```python
from build123d import *

# Parameters (mm, degrees)
F0_W      = 25.4
F0_H      = 76.2
F3_R      = 6.35
F4_DEPTH  = 50.8
F5_R      = 76.2
F7_R      = 152.4
F10_DEPTH = 25.4
F11_COUNT = 4


with BuildPart() as f1:
    # F0 (on Front) → F1 (revolve)
    with BuildSketch(Plane.XZ):
        with Locations((-139.7, 63.5)):
            Rectangle(F0_W, F0_H)
        Polygon((-152.4, 0), (0, 0), (0, 25.4), (-127, 25.4), (-152.4, 25.4), align=None)
    revolve(axis=Axis((0, 0, 12.7), (0, 0, 1)))

    # F3 (on offset) → F4 (cut)
    with BuildSketch(Plane.XZ.offset(152.4)):
        with Locations((0, 50.8)):
            Circle(F3_R)
    extrude(amount=-F4_DEPTH, mode=Mode.SUBTRACT)

    # F5 (on face) → F8 section 0
    with BuildSketch(Plane(origin=(0, 0, 0), x_dir=(1, 0, 0), z_dir=(0, 0, -1))):
        Circle(F5_R)
    # F7 (on offset) → F8 section 1
    with BuildSketch(Plane(origin=(0, 0, -152.4), x_dir=(1, 0, 0), z_dir=(0, 0, -1))):
        Circle(F7_R)
    loft()



with BuildPart() as f10:
    # F9 (on Right) → F10 (new body, symmetric)
    with BuildSketch(Plane.YZ):
        Polygon((177.8, -152.4), (25.4, -152.4), (54.7293936748, -203.2), (148.4706063252, -203.2), (207.1293936748, -304.8), (265.7881810245, -304.8), align=None)
    extrude(amount=F10_DEPTH, both=True)


with BuildPart() as f1_1:
    add(f1.part)

    add(f10.part)  # F11 merges F10
    # F11: F10 ×4 about axis
    f11_axis = Axis((0, 0, 0), (0, 0, -1))
    for i in range(1, F11_COUNT):
        add(f10.part.rotate(f11_axis, i * 360 / F11_COUNT))


solid = f1_1.part
```
The listing builds one solid part. Answer for the finished solid, in the listing's coordinates (mm). A direction names the side the tool comes from. Give positions to 0.01 mm unless a question says otherwise; leave off trailing zeros. Order: outer loops, then holes, each group sorted by start corner. A loop starts at its lowest first (then second) coordinate and runs counter-clockwise, first axis right, second up. Notation, with made-up numbers: M -21,-22 L -1,-22 A19 cw -1,-8 Z; hole C -30.5,-12 d9. An arc over 180 degrees is marked long. Put each result on its own line as item: value. Start each with the question number.
Item 1: Find the intervals of material crossed by line 1 along X through (y, z) = (0, 81); line 2 along Z through (x, y) = (0, -134.75); line 3 along Z through (x, y) = (0, -131.75), in increasing order.
Item 2: Which of the six approach directions +Z, -Z, +X, -X, +Y, -Y give full straight-line access (tool end or side, diameter ignored) to faces 5 (the face through (177.39, -0.36, -253.29)), 6 (the face through (0, -101, -203.2)), 7 (the face through (-2, -2, 25.4))?
Item 3: The part is cut by section A-A, the plane z = -270.5. Determine the outline of the cut face in (x, y), and give its area (3 significant figures).
Item 4: Flat-ended cylindrical pins translate along their axes: P1, Ø2, axis at y = -168, z = -177, coming from the +X side; P2, Ø12, axis at x = -6.5, z = -45, coming from the -Y side; P3, Ø8.5, axis at x = -9.5, y = -165.5, coming from the +Z side. Find the tip coordinate at first contact, or state that the pin passes through.
Item 5: The part is cut by section B-B, the plane y = 170. Determine the outline of the cut face in (x, z), and give its area (3 significant figures).
Item 6: For a pull along Z with two mould halves and no side action, classify faces 1 (the face through (-154, -25.4, -206)), 2 (the face through (-222.41, 0.36, -229.67)), 3 (the face through (82.614, 34.254, -26.467)), 4 (the face through (-75, 73, -152.4)) as +Z half, -Z half, draft (parallel to the pull), parting line (faces both ways), or undercut.
Answer key:
1. line 1: x = -152.4 to -127, 127 to 152.4
1. line 2: z = -203.2 to -117.1, 0 to 44.45, 57.15 to 101.6
1. line 3: z = -203.2 to -111.1, 0 to 44.45, 57.15 to 101.6
2. face 5: -Z, +Y, -Y
2. face 6: -Z, +X, -X
2. face 7: +Z
3. outline: M -245.99,-25.4 L -187.33,-25.4 L -187.33,25.4 L -245.99,25.4 Z; M -25.4,-245.99 L 25.4,-245.99 L 25.4,-187.33 L -25.4,-187.33 Z; M -25.4,187.33 L 25.4,187.33 L 25.4,245.99 L -25.4,245.99 Z; M 187.33,-25.4 L 245.99,-25.4 L 245.99,25.4 L 187.33,25.4 Z
3. area: 11,900 mm²
4. P1: stops at x = 25.4
4. P2: stops at y = -101.51
4. P3: stops at z = -152.4
5. outline: M -25.4,-240.49 L 25.4,-240.49 L 25.4,-152.4 L -25.4,-152.4 Z
5. area: 4,470 mm²
6. face 1: draft
6. face 2: +Z half
6. face 3: undercut
6. face 4: -Z half
